```python
from build123d import *

# Parameters (mm, degrees)
SKETCH_2_W               = 109.92
SKETCH_2_H               = 76
EXTRUDE_1_DEPTH          = 10
CUT_EXTRUDE_1_DEPTH      = 5
SKETCH_4_R               = 2
CUT_EXTRUDE_2_DEPTH      = 92.808295873
SKETCH_5_W               = 109.92
SKETCH_5_H               = 6
EXTRUDE_2_DEPTH          = 28.5
SKETCH_6_W               = 15
SKETCH_6_H               = 64
EXTRUDE_3_DEPTH          = 6.5
CUT_EXTRUDE_3_DEPTH      = 105.577891178
CUT_EXTRUDE_3_DEPTH_BACK = 105.577891178
SKETCH_7_R               = 2.1
SKETCH_9_R               = 2.1
CUT_EXTRUDE_4_DEPTH      = 95.274934055
CUT_EXTRUDE_5_DEPTH      = 5
FILLET_1_R               = 2


with BuildPart() as part:
    # 草圖2 → 填料-伸長1 (new body)
    with BuildSketch(Plane.XY):
        with Locations((12.52544527, 24.044160626)):
            Rectangle(SKETCH_2_W, SKETCH_2_H)
    extrude(amount=EXTRUDE_1_DEPTH)

    # 草圖3 → 除料-伸長1 (cut)
    with BuildSketch(Plane.XY.offset(10)):
        with BuildLine():
            Line((67.48544527, -6.055839374), (67.48544527, 54.144160626))
            Line((67.48544527, 54.144160626), (61.24181631, 50.538464901))
            ThreePointArc((61.24181631, 50.538464901), (61.408690367, 50.105080914), (61.46544527, 49.644160626))
            ThreePointArc((61.46544527, 49.644160626), (60.088104264, 47.81746208), (57.95299519, 48.639170705))
            Line((57.95299519, 48.639170705), (55.48544527, 47.214160626))
            Line((55.48544527, 47.214160626), (55.48544527, 0.874160626))
            Line((55.48544527, 0.874160626), (57.95299519, -0.550849453))
            ThreePointArc((57.95299519, -0.550849453), (60.088104264, 0.270859171), (61.46544527, -1.555839374))
            ThreePointArc((61.46544527, -1.555839374), (61.408690367, -2.016759663), (61.24181631, -2.45014365))
            Line((61.24181631, -2.45014365), (67.48544527, -6.055839374))
        make_face()
    extrude(amount=-CUT_EXTRUDE_1_DEPTH, mode=Mode.SUBTRACT)

    # 草圖4 → 除料-伸長2 (cut, through all)
    with BuildSketch(Plane.XY.offset(5)):
        with Locations((59.56544527, 41.644160626)):
            Circle(SKETCH_4_R)
        with Locations((59.56544527, 33.644160626)):
            Circle(SKETCH_4_R)
        with Locations((59.56544527, 6.444160626)):
            Circle(SKETCH_4_R)
        with Locations((59.56544527, 14.444160626)):
            Circle(SKETCH_4_R)
    extrude(amount=-CUT_EXTRUDE_2_DEPTH, mode=Mode.SUBTRACT)

    # 草圖5 → 填料-伸長2 (add)
    with BuildSketch(Plane.XY.offset(10)):
        with Locations((12.52544527, -10.955839374)):
            Rectangle(SKETCH_5_W, SKETCH_5_H)
        with Locations((12.52544527, 59.044160626)):
            Rectangle(SKETCH_5_W, SKETCH_5_H)
    extrude(amount=EXTRUDE_2_DEPTH)

    # 草圖6 → 填料-伸長3 (add)
    with BuildSketch(Plane.XY.offset(10)):
        with Locations((-34.93455473, 24.044160626)):
            Rectangle(SKETCH_6_W, SKETCH_6_H)
    extrude(amount=EXTRUDE_3_DEPTH)

    # 草圖7 → 除料-伸長3 (cut, two sides: drawn at the far end of the back side and taken through both)
    with BuildSketch(Plane(origin=(0, -7.955839374, 0), x_dir=(1, 0, 0), z_dir=(0, 1, 0)).offset(-CUT_EXTRUDE_3_DEPTH_BACK)):
        with Locations(Location((-36.43455473, -24.5, 0), (0, 0, 270))):
            Circle(SKETCH_7_R)
        with Locations(Location((-36.43455473, -32.5, 0), (0, 0, 270))):
            Circle(SKETCH_7_R)
    extrude(amount=CUT_EXTRUDE_3_DEPTH + CUT_EXTRUDE_3_DEPTH_BACK, mode=Mode.SUBTRACT)

    # 草圖9 → 除料-伸長4 (cut, through all)
    with BuildSketch(Plane.XY.offset(16.5)):
        with Locations((-36.43455473, 0.044160626)):
            Circle(SKETCH_9_R)
        with Locations((-36.43455473, 8.044160626)):
            Circle(SKETCH_9_R)
        with Locations((-36.43455473, 16.044160626)):
            Circle(SKETCH_9_R)
        with Locations((-36.43455473, 24.044160626)):
            Circle(SKETCH_9_R)
        with Locations((-36.43455473, 32.044160626)):
            Circle(SKETCH_9_R)
        with Locations((-36.43455473, 40.044160626)):
            Circle(SKETCH_9_R)
        with Locations((-36.43455473, 48.044160626)):
            Circle(SKETCH_9_R)
    extrude(amount=-CUT_EXTRUDE_4_DEPTH, mode=Mode.SUBTRACT)

    # 草圖10 → 除料-伸長5 (cut)
    with BuildSketch(Plane(origin=(0, 0, 0), x_dir=(-1, 0, 0), z_dir=(0, 0, -1))):
        with BuildLine():
            Line((32.43455473, 0.044160626), (32.43455473, 48.044160626))
            ThreePointArc((32.43455473, 48.044160626), (36.43455473, 52.044160626), (40.43455473, 48.044160626))
            Line((40.43455473, 48.044160626), (40.43455473, 0.044160626))
            ThreePointArc((40.43455473, 0.044160626), (36.43455473, -3.955839374), (32.43455473, 0.044160626))
        make_face()
    extrude(amount=-CUT_EXTRUDE_5_DEPTH, mode=Mode.SUBTRACT)

    # 圓角1
    fillet_1_edges = [part.edges().sort_by_distance(p)[0] for p in [
        (-27.43455473, 24.044160626, 16.5),
        (-27.43455473, 24.044160626, 10),
        (20.02544527, 56.044160626, 10),
        (20.02544527, -7.955839374, 10),
        (-42.43455473, 62.044160626, 19.25),
        (-42.43455473, -13.955839374, 19.25),
        (-42.43455473, 24.044160626, 0),
        (12.52544527, -13.955839374, 0),
        (12.52544527, 62.044160626, 0),
    ]]
    fillet(fillet_1_edges, radius=FILLET_1_R - 0.0001)  # a hair under: the kernel refuses the full size


solid = part.part
```
For this review, take the finished solid that the model builds, in its own axes (mm). A direction names the side the tool comes from. Round coordinates to 2 decimals unless told otherwise and drop trailing zeros. Loops run counter-clockwise (first coordinate to the right, second up) from the corner with the lowest first, then second, coordinate; pieces in that order, holes last.
(1) Wall thickness on line 1 along Y through (x, z) = (15.5, 32); line 2 along X through (y, z) = (60.2, 24.5); line 3 along X through (y, z) = (45.5, 2): over which ranges is each line inside the solid? List them lowest first.
Returned:
line 1: y = -13.96 to -7.96, 56.04 to 62.04
line 2: x = -42.43 to -38.53, -34.33 to 67.49
line 3: x = -42.43 to -40.43, -32.43 to 67.49
(2) We need section A-A (z = 36). Give the boundary of the cut face in (x, y), plus the area to 3 significant figures.
Returned:
outline: (-42.43, -11.96) arc R2 ccw to (-40.43, -13.96) - (67.49, -13.96) - (67.49, -7.96) - (-42.43, -7.96) - close; (-42.43, 56.04) - (67.49, 56.04) - (67.49, 62.04) - (-40.43, 62.04) arc R2 ccw to (-42.43, 60.04) - close
area: 1,320 mm2
(3) We need section C-C (x = -11). Give the boundary of the cut face in (y, z).
Returned:
outline: (-13.96, 2) arc R2 ccw to (-11.96, 0) - (60.04, 0) arc R2 ccw to (62.04, 2) - (62.04, 38.5) - (56.04, 38.5) - (56.04, 12) arc R2 cw to (54.04, 10) - (-5.96, 10) arc R2 cw to (-7.96, 12) - (-7.96, 38.5) - (-13.96, 38.5) - close
(4) Tool access review of faces 1 (the flat face through (55.485, 24, 8)), 2 (the flat face through (-32.435, 24, 2)), 3 (the cylindrical face through (-34.43, 8.67, 10.83)): name each direction out of +Z, -Z, +X, -X, +Y, -Y from which nothing blocks a thin tool from reaching the whole face with its end or side.
Returned:
face 1: +Z, +X
face 2: -Z
face 3: +Z, -Z
(5) Mouldability with a two-part tool opening along X and no side actions: class faces 4 (the flat face through (-42.435, 24, 12)), 5 (the cylindrical face through (60.49, 31.87, 2.54)), 6 (the flat face through (-27.435, 24, 13)) as released by +X, released by -X, zero draft, split by the parting line, or undercut.
Returned:
face 4: released by -X
face 5: undercut
face 6: released by +X
(6) We need section B-B (z = 24.5). Give the boundary of the cut face in (x, y), plus the area to 3 significant figures.
Returned:
outline: (-42.43, -11.96) arc R2 ccw to (-40.43, -13.96) - (-38.53, -13.96) - (-38.53, -7.96) - (-42.43, -7.96) - close; (-42.43, 56.04) - (-38.53, 56.04) - (-38.53, 62.04) - (-40.43, 62.04) arc R2 ccw to (-42.43, 60.04) - close; (-34.33, -13.96) - (67.49, -13.96) - (67.49, -7.96) - (-34.33, -7.96) - close; (-34.33, 56.04) - (67.49, 56.04) - (67.49, 62.04) - (-34.33, 62.04) - close
area: 1,270 mm2
(7) Clearance check with flat-ended pins moving along their axes: P1, Ø10, axis at x = -22, y = 11.5, coming from the +Z side; P2, Ø4, axis at x = -38.5, y = 22, coming from the +Z side; P3, Ø3.5, axis at x = 61, y = 18, coming from the +Z side. State where each tip first meets the part, or that it passes through.
Returned:
P1: stops at z = 10.76
P2: stops at z = 16.5
P3: stops at z = 5
(8) We need section D-D (z = 7). Give the boundary of the cut face in (x, y), plus the area to 3 significant figures.
Returned:
outline: (-42.43, -11.96) arc R2 ccw to (-40.43, -13.96) - (67.49, -13.96) - (67.49, -6.06) - (61.24, -2.45) arc R1.9 ccw to (57.95, -0.55) - (55.49, 0.87) - (55.49, 47.21) - (57.95, 48.64) arc R1.9 ccw to (61.24, 50.54) - (67.49, 54.14) - (67.49, 62.04) - (-40.43, 62.04) arc R2 ccw to (-42.43, 60.04) - close; hole circle Ø4.2 at (-36.43, 0.04); hole circle Ø4.2 at (-36.43, 8.04); hole circle Ø4.2 at (-36.43, 16.04); hole circle Ø4.2 at (-36.43, 24.04); hole circle Ø4.2 at (-36.43, 32.04); hole circle Ø4.2 at (-36.43, 40.04); hole circle Ø4.2 at (-36.43, 48.04)
area: 7,630 mm2
